Autodesk Inventor part; units mm, degrees
ref_plane "YZ Plane" through (0, 0, 0) normal (1, 0, 0) x (0, 1, 0)
ref_plane "XZ Plane" through (0, 0, 0) normal (0, 1, 0) x (-1, 0, 0)
ref_plane "XY Plane" through (0, 0, 0) normal (0, 0, 1) x (1, 0, 0)
sketch "Sketch1" plane through (0, 0, 0) normal (0, 1, 0) x (-1, 0, 0)
  line L0 (0, 0) -> (809, 0)
  line L1 (809, 0) -> (809, -50)
  line L2 (809, -50) -> (0, -50)
  line L3 (0, -50) -> (0, 0)
  dimension "d0" = 809
  dimension "d1" = 50
extrude "Extrusion1" add sketch "Sketch1" along normal blind 3
sketch "Sketch2" plane through (0, 0, 0) normal (0, -1, 0) x (1, 0, 0)
  line L0 (-806, -3) -> (-3, -3)
  line L1 (-3, -3) -> (-3, -47)
  line L2 (-3, -47) -> (-806, -47)
  line L3 (-806, -47) -> (-806, -3)
  line L4 (-809, 0) -> (0, 0)
  line L5 (-809, 0) -> (-809, -50)
  line L6 (-206, -3) -> (-203, -3)
  line L7 (-203, -3) -> (-203, -47)
  line L8 (-203, -47) -> (-206, -47)
  line L9 (-206, -47) -> (-206, -3)
  line L10 (0, -50) -> (-809, -50)
  line L11 (-809, 0) -> (0, 0)
  line L12 (0, 0) -> (0, -50)
  line L13 (0, -50) -> (-809, -50)
  line L14 (-809, -50) -> (-809, 0)
  dimension "d4" = 803
  dimension "d5" = 44
  dimension "d6" = 3
  dimension "d7" = 3
  dimension "d8" = 3
  dimension "d9" = 600
extrude "Extrusion2" add sketch "Sketch2" along normal blind 12.5 and the other way blind 12.5 contours L0 L7 L2 L9 | L4 L12 L10 L5
sketch "Sketch3" plane through (0, -12.5, 0) normal (0, -1, 0) x (1, 0, 0)
  line L0 (0, 0) -> (-809, 0)
  line L1 (0, -50) -> (-809, -50)
  line L2 (-229.5, 0) -> (-179.5, 0)
  line L3 (-179.5, 0) -> (-179.5, -50)
  line L4 (-179.5, -50) -> (-229.5, -50)
  line L5 (-229.5, -50) -> (-229.5, 0)
  line L6 (-203, -47) -> (-203, -3)
  line L7 (-809, 0) -> (0, 0)
  line L8 (-269.5, 0) -> (-284.5, 0)
  line L9 (-284.5, 0) -> (-284.5, -50)
  line L10 (-284.5, -50) -> (-269.5, -50)
  line L11 (-269.5, -50) -> (-269.5, 0)
  line L12 (-809, -50) -> (0, -50)
  line L13 (-284.5, 0) -> (-287.5, 0)
  line L14 (-287.5, 0) -> (-287.5, -50)
  line L15 (-287.5, -50) -> (-284.5, -50)
  line L16 (-284.5, -50) -> (-284.5, 0)
  line L17 (-287.5, 0) -> (-302.5, 0)
  line L18 (-302.5, 0) -> (-302.5, -50)
  line L19 (-302.5, -50) -> (-287.5, -50)
  line L20 (-287.5, -50) -> (-287.5, 0)
  dimension "d14" = 50
  dimension "d15" = 23.5
  dimension "d18" = 15
  dimension "d19" = 40
  dimension "d24" = 3
  dimension "d25" = 15
  dimension "d26" = 50
extrude "Extrusion3" add sketch "Sketch3" along normal blind 3 contours L3 L1 L5 L0 | L11 L1 L9 L0 | L14 L1 L18 L0
sketch "Sketch4" plane through (0, 0, 0) normal (0, -1, 0) x (1, 0, 0)
  line L0 (-284.5, -3) -> (-284.5, -47)
  line L1 (-284.5, -3) -> (-287.5, -3)
  line L2 (-287.5, -3) -> (-287.5, -47)
  line L3 (-287.5, -47) -> (-284.5, -47)
  line L4 (-284.5, -47) -> (-284.5, -3)
  point P0 (0, 0)
  dimension "d20" = 3
  dimension "d21" = 44
extrude "Extrusion4" add sketch "Sketch4" along normal blind 50
properties part number "Boom" material "Wood (Birch)"
Could you check a few things on this model? Use its own coordinates, in mm. A direction names the side the tool comes from. Give positions to 0.01 mm unless a question says otherwise; leave off trailing zeros. Write each loop counter-clockwise with the first axis right and the second up, starting at its lowest first coordinate (ties: lowest second). Pieces come first, ordered by that corner, then holes. Notation, with made-up numbers: (-11, -30) -> (39, -30) arc R26 ccw to (39, -10) -> close; hole circle Ø7 at (-16.5, -23.5). An arc over 180 degrees is marked (long way). Write each question's results on one line, items separated by ' | '. Start each with the question number.
Q1. Which directions (+Z, -Z, +X, -X, +Y, -Y) give clear straight access to the entire face, cutting with the end or side of a thin tool? Please do faces 1 (the face through (-806, -6, -25)), 2 (the face through (-287.5, -33, -25)), 3 (the face through (-246, -6, -3)), 4 (the face through (-284.5, -33, -25)).
Q2. Suppose I cut it at B-B, the plane y = -34. List the corners of the cut face in (x, z) for me.
Q3. Suppose I cut it at A-A, the plane x = -532.5. List the corners of the cut face in (y, z) for me, and give its area (3 significant figures).
Q4. I'm going to push flat-ended pins straight in: pin 1 Ø16.5 at (x, z) = (-294.5, -21.5) entering from +Y; pin 2 Ø3.5 at (x, y) = (-286, -38.5) entering from -Z; pin 3 Ø3 at (y, z) = (-37.5, -14.5) entering from +X. Where does each tip first touch, or does it pass through?
Q5. I need wall thicknesses on probe 1 along X at (y, z) = (-15, -11); probe 2 along Z at (x, y) = (-149.5, 5.5); probe 3 along X at (y, z) = (-41.5, -16.5). Which ranges of each line are inside material? Lowest first, please.
Q6. We'd pull the mould along X, two halves only. Please class faces 5 (the face through (-809, 0, -25)), 6 (the face through (-102, 0, -25)), 7 (the face through (-410, -2, -50)): +X half, -X half, draft (parallel to the pull), parting line (faces both ways), or undercut.
Outcome:
1) face 1: -Y | face 2: +Z, -Z, -X, -Y | face 3: none | face 4: +Z, -Z, +X, -Y
2) outline: (-287.5, -47) -> (-284.5, -47) -> (-284.5, -3) -> (-287.5, -3) -> close
3) outline: (-12.5, -50) -> (12.5, -50) -> (12.5, -47) -> (3, -47) -> (3, -3) -> (12.5, -3) -> (12.5, 0) -> (-12.5, 0) -> (-12.5, -3) -> (0, -3) -> (0, -47) -> (-12.5, -47) -> close | area: 282 mm2
4) pin 1: y = 3 | pin 2: z = -47 | pin 3: x = -284.5
5) probe 1: -302.5 to -269.5, -229.5 to -179.5 | probe 2: -50 to -47, -3 to 0 | probe 3: -287.5 to -284.5
6) face 5: -X half | face 6: undercut | face 7: draft
